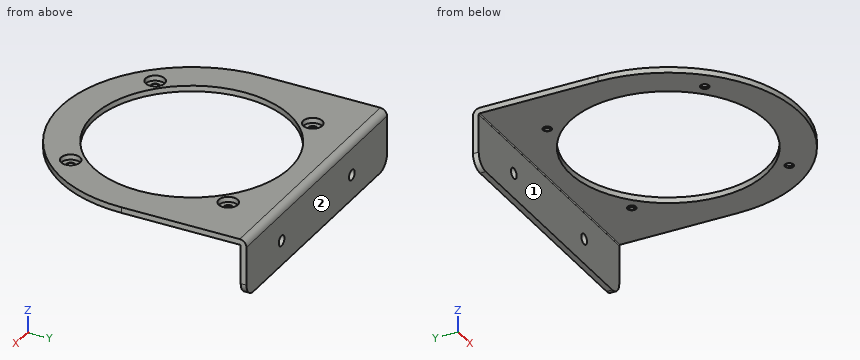
```python
from build123d import *

# Parameters (mm, degrees)
BASE_FLANGE1_DEPTH           = 4.365
EDGE_FLANGE1_STRIP_W         = 18.9332
EDGE_FLANGE1_STRIP_H         = 4.365
EDGE_FLANGE1_STRIP_CUT_DEPTH = 200
EDGE_FLANGE1_DEPTH           = 200
SKETCH10_R                   = 75
CUT_EXTRUDE1_DEPTH           = 10
FILLET1_R                    = 10
SKETCH12_R                   = 4
CUT_EXTRUDE3_DEPTH           = 10
CIRPATTERN1_COUNT            = 4


# Sheet-metal steps are written as plain solids
with BuildPart() as part:
    # Sketch2 → Base-Flange1 (new body)
    with BuildSketch(Plane.XY):
        with BuildLine():
            Line((-100, 0), (-100, 95.4))
            Line((-100, 95.4), (100, 95.4))
            Line((100, 95.4), (100, 0))
            ThreePointArc((100, 0), (0, -100), (-100, 0))
        make_face()
    extrude(amount=-BASE_FLANGE1_DEPTH)

    # Edge-Flange1 strip (across the edge) → Edge-Flange1 strip cut (cut)
    with BuildSketch(Plane(origin=(-100, 95.4, -4.365), x_dir=(0, -1, 0), z_dir=(1, 0, 0))):
        with Locations((-4.365, -2.1825)):
            Rectangle(EDGE_FLANGE1_STRIP_W, EDGE_FLANGE1_STRIP_H)
    extrude(amount=EDGE_FLANGE1_STRIP_CUT_DEPTH, mode=Mode.SUBTRACT)

    # Edge-Flange1 section (across the edge) → Edge-Flange1 (add)
    with BuildSketch(Plane(origin=(-100, 95.4, -4.365), x_dir=(0, -1, 0), z_dir=(1, 0, 0))):
        with BuildLine():
            Line((0, 0.7366), (0, 40))
            Line((0, 40), (4.365, 40))
            Line((4.365, 40), (4.365, 0.7366))
            ThreePointArc((4.365, 0.7366), (4.580745145, 0.215745145), (5.1016, 0))
            Line((5.1016, 0), (5.1016, -4.365))
            ThreePointArc((5.1016, -4.365), (1.494224045, -2.870775955), (0, 0.7366))
        make_face()
    extrude(amount=EDGE_FLANGE1_DEPTH)

    # Sketch10 → Cut-Extrude1 (cut)
    with BuildSketch(Plane.XY):
        Circle(SKETCH10_R)
    extrude(amount=-CUT_EXTRUDE1_DEPTH, mode=Mode.SUBTRACT)

    # Fillet1
    fillet1_edges = [part.edges().sort_by_distance(p)[0] for p in [
        (-100, 93.2175, -44.365),
        (100, 93.2175, -44.365),
    ]]
    fillet(fillet1_edges, radius=FILLET1_R)

    # Sketch12 → Cut-Extrude3 (cut)
    with BuildSketch(Plane(origin=(0, 95.4, 0), x_dir=(1, 0, 0), z_dir=(0, 1, 0))):
        with Locations(Location((-50, 25.365, 0), (0, 0, 270))):
            Circle(SKETCH12_R)
        with Locations(Location((50, 25.365, 0), (0, 0, 90))):
            Circle(SKETCH12_R)
    extrude(amount=-CUT_EXTRUDE3_DEPTH, mode=Mode.SUBTRACT)

    # Sketch14 → CBORE for M6 Hex Head Screw1 (revolve, cut)
    with BuildSketch(Plane(origin=(-60.104076401, 60.104076401, 0), x_dir=(0, -1, 0), z_dir=(1, 0, 0))):
        Polygon((0, 0), (0, 44.365), (3.3, 44.365), (3.3, 4), (7.2735, 4), (7.2735, 0.025), (7.2985, 0), align=None)
    cbore_for_m6_hex_head_screw1 = revolve(axis=Axis((-60.104076401, 60.104076401, 6.35), (0, 0, -1)), mode=Mode.SUBTRACT)

    # CirPattern1: CBORE for M6 Hex Head Screw1 ×4 about axis
    cirpattern1_axis = Axis((0, 0, 0), (0, 0, 1))
    for i in range(1, CIRPATTERN1_COUNT):
        add(cbore_for_m6_hex_head_screw1.rotate(cirpattern1_axis, i * 360 / CIRPATTERN1_COUNT), mode=Mode.SUBTRACT)


solid = part.part
```
Source: CAD feature listing. Evaluate the final solid. Frame: model axes, mm. Face numbers are marked on the shaded views. A direction names the side the tool comes from. Round coordinates to 2 decimals unless told otherwise and drop trailing zeros. Loops run counter-clockwise (first coordinate to the right, second up) from the corner with the lowest first, then second, coordinate; pieces in that order, holes last. Notation, with made-up numbers: M -9.5,-36 L 30.5,-36 A17 ccw 30.5,-6 Z; hole C 70.5,35 d9. An arc over 180 degrees is marked long. Put each result on its own line as item: value.
(1) Access query for the marked faces 1 and 2. Directions: +Z, -Z, +X, -X, +Y, -Y. A direction counts if a zero-diameter tool reaches every point of the face in a straight line with its end or side. Return the directions, or none.
Solutions:
face 1: -Z, +X, -X, -Y
face 2: +Z, -Z, +X, -X, +Y
(2) Section B-B, the plane x = 50. Return loops of the section in (y, z) (3 decimals), and give its area (3 significant figures).
Solutions:
outline: M -86.603,-4.365 L -55.902,-4.365 L -55.902,0 L -86.603,0 Z; M 55.902,-4.365 L 90.298,-4.365 A0.737 cw 91.035,-5.102 L 91.035,-21.365 L 95.4,-21.365 L 95.4,-5.102 A5.102 ccw 90.298,0 L 55.902,0 Z; M 91.035,-44.365 L 95.4,-44.365 L 95.4,-29.365 L 91.035,-29.365 Z
area: 441 mm²
(3) Section D-D, the plane x = -79.5. Return loops of the section in (y, z) (3 decimals).
Solutions:
outline: M -60.661,-4.365 L 90.298,-4.365 A0.737 cw 91.035,-5.102 L 91.035,-44.365 L 95.4,-44.365 L 95.4,-5.102 A5.102 ccw 90.298,0 L -60.661,0 Z
(4) Section A-A, the plane x = 0. Return loops of the section in (y, z) (3 decimals), and give its area (3 significant figures).
Solutions:
outline: M -100,-4.365 L -75,-4.365 L -75,0 L -100,0 Z; M 75,-4.365 L 90.298,-4.365 A0.737 cw 91.035,-5.102 L 91.035,-44.365 L 95.4,-44.365 L 95.4,-5.102 A5.102 ccw 90.298,0 L 75,0 Z
area: 367 mm²
(5) Section C-C, the plane y = -34.5. Return loops of the section in (x, z) (3 decimals), and give its area (3 significant figures).
Solutions:
outline: M -93.86,-4.365 L -66.594,-4.365 L -66.594,0 L -93.86,0 Z; M 66.594,-4.365 L 93.86,-4.365 L 93.86,0 L 66.594,0 Z
area: 238 mm²
(6) Ray query, line 1 (Y direction, x = -7.5, z = -5); line 2 (Z direction, x = 6, y = -92) (3 decimals); line 3 (Y direction, x = 0, z = -1.6). Return the intervals inside material, ascending. Write a range as [from, to].
Solutions:
line 1: [91.03, 95.4]
line 2: [-4.365, 0]
line 3: [-100, -75], [75, 94.01]
(7) First-contact query: pin 1 (11.5 mm diameter, centred on x = 61, y = -60, fed in from +Z); pin 2 (5 mm diameter, centred on x = -31, z = -37.5, fed in from -Y) (3 decimals). Flat tips, straight axial feed; report the tip coordinate or a pass-through.
Solutions:
pin 1: z = -4
pin 2: y = 91.035
